from build123d import *

# Parameters (mm, degrees)
SKETCH2_R                      = 1.4
BOSS_EXTRUDE1_DEPTH            = 10
SKETCH3_R                      = 3
SKETCH3_R_2                    = 1.4
BOSS_EXTRUDE2_DEPTH            = 2.54
CBORE_FOR_M5_SHCS1_D           = 5.5
CBORE_FOR_M5_SHCS1_DEPTH       = 12
CBORE_FOR_M5_SHCS1_CBORE_D     = 10
CBORE_FOR_M5_SHCS1_CBORE_DEPTH = 5
CBORE_FOR_M5_SHCS1_TIP         = 1.652366702


with BuildPart() as part:
    # Sketch2 → Boss-Extrude1 (new body)
    with BuildSketch(Plane(origin=(0, 0, 0), x_dir=(1, 0, 0), z_dir=(0, 1, 0))):
        with BuildLine():
            Line((-40.8, 14.5), (-39, 14.5))
            Line((-39, 14.5), (-39, -14.5))
            Line((-39, -14.5), (-40.8, -14.5))
            ThreePointArc((-40.8, -14.5), (-50.8, -24.5), (-40.8, -34.5))
            Line((-40.8, -34.5), (-19, -34.5))
            Line((-19, -34.5), (-19, 34.5))
            Line((-19, 34.5), (-40.8, 34.5))
            ThreePointArc((-40.8, 34.5), (-50.8, 24.5), (-40.8, 14.5))
        make_face()
        with Locations(Location((-29, -24.5, 0), (0, 0, 270))):
            Circle(SKETCH2_R, mode=Mode.SUBTRACT)
        with Locations(Location((-29, 24.5, 0), (0, 0, 270))):
            Circle(SKETCH2_R, mode=Mode.SUBTRACT)
    extrude(amount=BOSS_EXTRUDE1_DEPTH)

    # Sketch3 → Boss-Extrude2 (add)
    # profile 1 of 2: a face of its own
    with BuildSketch(Plane(origin=(0, 10, 0), x_dir=(1, 0, 0), z_dir=(0, 1, 0))):
        with Locations(Location((-29, 24.5, 0), (0, 0, 90))):
            Circle(SKETCH3_R)
        with Locations(Location((-29, 24.5, 0), (0, 0, 270))):
            Circle(SKETCH3_R_2, mode=Mode.SUBTRACT)
    # profile 2 of 2: a face of its own
    with BuildSketch(Plane(origin=(0, 10, 0), x_dir=(1, 0, 0), z_dir=(0, 1, 0))):
        with Locations(Location((-29, -24.5, 0), (0, 0, 90))):
            Circle(SKETCH3_R)
        with Locations(Location((-29, -24.5, 0), (0, 0, 270))):
            Circle(SKETCH3_R_2, mode=Mode.SUBTRACT)
    extrude(amount=BOSS_EXTRUDE2_DEPTH)

    # CBORE for M5 SHCS1
    with Locations(Plane(origin=(0, 10, 0), x_dir=(1, 0, 0), z_dir=(0, 1, 0))):
        with Locations((-40.8, -24.5), (-40.8, 24.5)):
            CounterBoreHole(CBORE_FOR_M5_SHCS1_D / 2, CBORE_FOR_M5_SHCS1_CBORE_D / 2, CBORE_FOR_M5_SHCS1_CBORE_DEPTH, depth=CBORE_FOR_M5_SHCS1_DEPTH)
            with Locations((0, 0, -(CBORE_FOR_M5_SHCS1_DEPTH + CBORE_FOR_M5_SHCS1_TIP / 2))):  # 118° drill point
                Cone(0, CBORE_FOR_M5_SHCS1_D / 2, CBORE_FOR_M5_SHCS1_TIP, mode=Mode.SUBTRACT)


solid = part.part
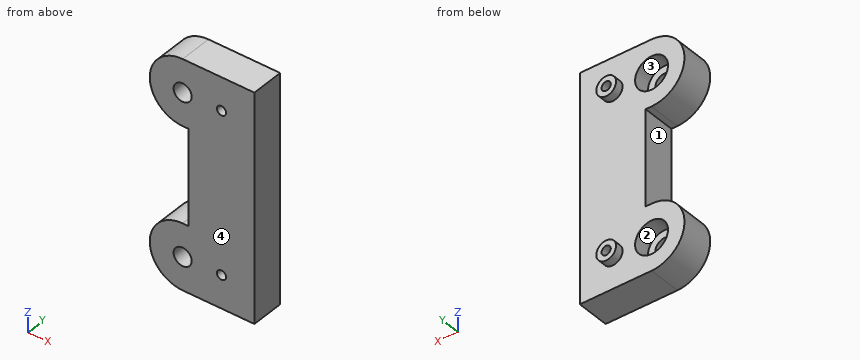
Build history of the part. All positions in model axes, mm. Face numbers are marked on the shaded views. Coordinates: 2 decimals unless noted, no trailing zeros. Write each loop counter-clockwise with the first axis right and the second up, starting at its lowest first coordinate (ties: lowest second). Pieces come first, ordered by that corner, then holes.
(1) Pin check, flat tips, straight feed: pin 1 Ø2 at (x, z) = (-36.5, 15) entering from +Y; pin 2 Ø1 at (y, z) = (3, 15) entering from -X; pin 3 Ø5 at (y, z) = (9, -21.5) entering from -X; pin 4 Ø3.5 at (x, z) = (-29, -24.5) entering from +Y. Stop position of each tip, or through.
(2) Cut at A-A on y = 3. List the corners of the cut face in (x, z), and give its area (3 significant figures).
(3) Drill centre lines: line 1 (Z direction, x = -40.8, y = 2.2); line 2 (X direction, y = 2.45, z = 24.5); line 3 (X direction, y = 8.95, z = -24.5). Where is each one in solid material? Low to high.
(4) Cut at C-C on x = -29. List the corners of the cut face in (y, z).
(5) Cut at D-D on y = 11.75. List the corners of the cut face in (x, z), and give its area (3 significant figures).
(6) Mould opens along X. For the marked faces 1, 2, 3 and 4 say: pulls with the +X half, pulls with the -X half, needs draft (parallel to the pull), parting line crosses it, or undercut.
(7) Cut at B-B on z = 24.5. List the corners of the cut face in (x, y), and give its area (3 significant figures).
Working result:
1. pin 1: stops at y = 10
1. pin 2: stops at x = -45.16
1. pin 3: stops at x = -50.79
1. pin 4: stops at y = 12.54
2. outline: (-40.8, -34.5) - (-19, -34.5) - (-19, 34.5) - (-40.8, 34.5) arc R10 ccw to (-40.8, 14.5) - (-39, 14.5) - (-39, -14.5) - (-40.8, -14.5) arc R10 ccw to start; hole circle Ø5.5 at (-40.8, -24.5); hole circle Ø5.5 at (-40.8, 24.5); hole circle Ø2.8 at (-29, -24.5); hole circle Ø2.8 at (-29, 24.5)
2. area: 1,710 mm2
3. line 1: z = -34.5 to -27.25, -21.75 to -14.5, 14.5 to 21.75, 27.25 to 34.5
3. line 2: x = -50.8 to -43.55, -38.05 to -30.4, -27.6 to -19
3. line 3: x = -50.8 to -45.8, -35.8 to -30.4, -27.6 to -19
4. outline: (0, -34.5) - (10, -34.5) - (10, -27.5) - (12.54, -27.5) - (12.54, -25.9) - (0, -25.9) - close; (0, -23.1) - (12.54, -23.1) - (12.54, -21.5) - (10, -21.5) - (10, 21.5) - (12.54, 21.5) - (12.54, 23.1) - (0, 23.1) - close; (0, 25.9) - (12.54, 25.9) - (12.54, 27.5) - (10, 27.5) - (10, 34.5) - (0, 34.5) - close
5. outline: circle Ø6 at (-29, -24.5); circle Ø6 at (-29, 24.5); hole circle Ø2.8 at (-29, -24.5); hole circle Ø2.8 at (-29, 24.5)
5. area: 44.2 mm2
6. face 1: pulls with the -X half
6. face 2: undercut
6. face 3: undercut
6. face 4: needs draft
7. outline: (-50.8, 0) - (-43.55, 0) - (-43.55, 5) - (-45.8, 5) - (-45.8, 10) - (-50.8, 10) - close; (-38.05, 0) - (-30.4, 0) - (-30.4, 12.54) - (-32, 12.54) - (-32, 10) - (-35.8, 10) - (-35.8, 5) - (-38.05, 5) - close; (-27.6, 0) - (-19, 0) - (-19, 10) - (-26, 10) - (-26, 12.54) - (-27.6, 12.54) - close
7. area: 221 mm2
